from build123d import *

# Parameters (mm, degrees)
SKETCH_1_R      = 13
SKETCH_1_R_2    = 8.5
EXTRUDE_1_DEPTH = 5
EXTRUDE_START   = -1.1
SKETCH_2_R      = 14
SKETCH_2_R_2    = 13
EXTRUDE_2_DEPTH = 1.1
FILLET_1_R      = 0.3
SKETCH_3_W      = 0.5
SKETCH_3_H      = 2.575


with BuildPart() as part:
    # 草图1 → 凸台-拉伸1 (new body)
    with BuildSketch(Plane.XY):
        Circle(SKETCH_1_R)
        Circle(SKETCH_1_R_2, mode=Mode.SUBTRACT)
    extrude(amount=EXTRUDE_1_DEPTH)

    # 草图2 → 凸台-拉伸2 (add)
    with BuildSketch(Plane.XY.offset(5).offset(EXTRUDE_START)):
        Circle(SKETCH_2_R)
        Circle(SKETCH_2_R_2, mode=Mode.SUBTRACT)
    extrude(amount=EXTRUDE_2_DEPTH)

    # 圆角1
    fillet_1_edges = [part.edges().sort_by_distance(p)[0] for p in [
        (-13, 0, 0),
    ]]
    fillet(fillet_1_edges, radius=FILLET_1_R)

    # 草图3 → 切除-旋转1 (revolve, cut)
    with BuildSketch(Plane(origin=(0, 0, 0), x_dir=(0, 0, -1), z_dir=(1, 0, 0)), mode=Mode.PRIVATE) as cut_revolve_1_sk:
        with Locations((-0.25, 10.7875)):
            Rectangle(SKETCH_3_W, SKETCH_3_H)
        with Locations((-4.75, 10.7875)):
            Rectangle(SKETCH_3_W, SKETCH_3_H)
    revolve(cut_revolve_1_sk.sketch.rotate(Axis((0, 0, 0), (0, 0, 1)), 90), axis=Axis((0, 0, 0), (0, 0, 1)), mode=Mode.SUBTRACT)


solid = part.part
Design review of the part built by this model. Coordinates are the model's own, in mm. A direction names the side the tool comes from. Give positions to 0.01 mm unless a question says otherwise; leave off trailing zeros. Loops run counter-clockwise (first coordinate to the right, second up) from the corner with the lowest first, then second, coordinate; pieces in that order, holes last. Notation, with made-up numbers: M -2.75,82.25 L 34.25,82.25 A14 cw 34.25,90.25 Z; hole C -12.5,8.25 d3. An arc over 180 degrees is marked long. Answer as a JSON object with one key per item and string values.
Item 1: Machinability: for faces 1 (the face through (12.932, -5.362, 4.442)), 2 (the face through (-8.1, 5.3, 4.5)), 3 (the face through (12.063, -0.531, 0.246)), which of the approach directions +Z, -Z, +X, -X, +Y, -Y give a long, thin tool a straight path to every point of the face, cutting with its end or side? Answer none if there is none.
Output values:
{"face 1": "+Z, -Z", "face 2": "+Z", "face 3": "-Z"}
Item 2: We need section C-C (z = 2.15). State the section outline as (x, y) points, and give its area (3 significant figures).
Output values:
{"outline": "C 0,0 d26; hole C 0,0 d17", "area": "304 mm2"}
Item 3: Mouldability with a two-part tool opening along Y and no side actions: class faces 4 (the face through (2.059, 9.274, 0.246)), 5 (the face through (-2.2, -8.4, 0)), 6 (the face through (-10.316, -7.91, 2.075)) as pulls with the +Y half, pulls with the -Y half, needs draft (parallel to the pull), parting line crosses it, or undercut.
Output values:
{"face 4": "undercut", "face 5": "needs draft", "face 6": "parting line crosses it"}
Item 4: For P1, Ø1.5, axis at x = -9, z = 4, coming from the +Y side; P2, Ø1.5, axis at y = 1.5, z = 2.5, coming from the -X side; P3, Ø2, axis at y = -1, z = 3, coming from the -X side; P4, Ø10, axis at x = 0, y = 0, coming from the +Z side, all flat-tipped, find the tip position at first contact; note any pin that passes through.
Output values:
{"P1": "stops at y = 11.31", "P2": "stops at x = -12.98", "P3": "stops at x = -13.99", "P4": "passes through"}
Item 5: Wall thickness on line 1 along Y through (x, z) = (0, 4.8) (3 decimals); line 2 along Y through (x, z) = (0, 2.05); line 3 along Y through (x, z) = (0, 4.05): over which ranges is each line inside the solid? List them lowest first.
Output values:
{"line 1": "y = -14 to -12.075, -9.5 to -8.5, 8.5 to 9.5, 12.075 to 14", "line 2": "y = -13 to -8.5, 8.5 to 13", "line 3": "y = -14 to -8.5, 8.5 to 14"}
